Autodesk Inventor part; units mm, degrees
ref_plane "YZ Plane" through (0, 0, 0) normal (1, 0, 0) x (0, 1, 0)
ref_plane "XZ Plane" through (0, 0, 0) normal (0, 1, 0) x (-1, 0, 0)
ref_plane "XY Plane" through (0, 0, 0) normal (0, 0, 1) x (1, 0, 0)
sketch "Sketch1" plane through (0, 0, 0) normal (0, 0, 1) x (1, 0, 0)
  line L0 (-11, 0) -> (11, 0)
  line L1 (11, 0) -> (11, 30)
  line L2 (11, 30) -> (-11, 0)
  point P0 (0, 0)
  point P1 (0, 0)
  dimension "d0" = 22
  dimension "d1" = 30
extrude "Extrusion1" add sketch "Sketch1" along normal mid plane 10
sketch "Sketch2" plane through (0, 0, 0) normal (0, 0, 1) x (1, 0, 0)
  line L0 (11, 30) -> (11, 0) construction
  line L1 (11, 0) -> (-11, 0) construction
  line L2 (-11, 0) -> (11, 30) construction
  line L3 (8.1, 8) -> (0, 8)
  line L4 (0, 8) -> (0, 5)
  line L5 (0, 5) -> (8.1, 5)
  line L6 (8.1, 5) -> (8.1, 8)
  line L7 (6, 11) -> (9, 11)
  line L8 (9, 11) -> (9, 19.1)
  line L9 (9, 19.1) -> (6, 19.1)
  line L10 (6, 19.1) -> (6, 11)
  point P0 (0, 0)
  point P1 (0, 6.5)
  point P2 (0, 0)
  point P3 (11, 15)
  dimension "d4" = 8.1
  dimension "d5" = 5
  dimension "d6" = 3
  dimension "d7" = 3
  dimension "d8" = 8.1
  dimension "d9" = 2
  dimension "d10" = 3
extrude "Extrusion2" cut sketch "Sketch2" along normal through all both and the other way through all
sketch "Sketch3" plane through (11, 0, 5) normal (1, 0, 0) x (0, 0, -1)
  line L0 (10, 19.1) -> (10, 11) construction
  line L1 (10, 19.1) -> (0, 19.1) construction
  line L2 (0, 11) -> (0, 19.1) construction
  line L3 (10, 11) -> (0, 11) construction
  line L4 (10, 19.1) -> (0, 19.1) construction
  line L5 (5, 19.1) -> (5, 11) construction
  line L6 (0, 15.05) -> (10, 15.05) construction
  line L7 (10, 19.1) -> (10, 11) construction
  circle A0 centre (5, 15.05) radius 2.75
  point P0 (5, 0)
  dimension "d13" = 5.5
extrude "Extrusion3" cut sketch "Sketch3" against normal up to surface (5 mm away)
sketch "Sketch4" plane through (-11, 0, 5) normal (0, -1, 0) x (1, 0, 0)
  line L0 (19.1, -10) -> (11, -10) construction
  line L1 (19.1, -10) -> (19.1, 0) construction
  line L2 (11, 0) -> (19.1, 0) construction
  line L3 (11, 0) -> (11, -10) construction
  line L4 (19.1, 0) -> (11, 0) construction
  line L5 (15.05, 0) -> (15.05, -10) construction
  line L6 (19.1, -10) -> (11, -10) construction
  line L7 (11, -5) -> (19.1, -5) construction
  circle A0 centre (15.05, -5) radius 2.75
  dimension "d16" = 5.5
extrude "Extrusion4" cut sketch "Sketch4" against normal up to surface (8 mm away)
properties part number "ligamento_obj4"
Geometry: final body of the model. Coordinates: model frame, mm. A direction names the side the tool comes from. Give positions to 0.01 mm unless a question says otherwise; leave off trailing zeros. Order: outer loops, then holes, each group sorted by start corner. A loop starts at its lowest first (then second) coordinate and runs counter-clockwise, first axis right, second up. Notation, with made-up numbers: (-15.75, -37) - (1.25, -37) arc R12 ccw to (1.25, -22) - close; hole circle Ø4 at (-5, -37). An arc over 180 degrees is marked (long way). Use CSV: the item, a comma, the result in double quotes.
1. Section query C-C (z = 4). Output: boundary loops of the cut face in (x, y), plus the area to 3 significant figures.
Answers below:
outline,"(-11, 0) - (11, 0) - (11, 30) - close; hole (0, 5) - (8.1, 5) - (8.1, 8) - (0, 8) - close; hole (6, 11) - (9, 11) - (9, 19.1) - (6, 19.1) - close"
area,"281 mm2"
2. Access query for faces 5 (the face through (11, 11, 0)), 6 (the face through (4, 8, 0)). Directions: +Z, -Z, +X, -X, +Y, -Y. A direction counts if a zero-diameter tool reaches every point of the face in a straight line with its end or side. Return the directions, or none.
Answers below:
face 5,"+Z, -Z, +X, +Y, -Y"
face 6,"+Z, -Z"
3. Mould query, pull axis Z, two halves, no side actions, for faces 1 (the face through (5, 9, 5)), 2 (the face through (6.59, 2.46, -1.05)), 3 (the face through (10.014, 12.365, 0.596)), 4 (the face through (0, 15, 0)). Classes: +Z half, -Z half, draft (parallel to the pull), parting line (faces both ways), or undercut.
Answers below:
face 1,"+Z half"
face 2,"undercut"
face 3,"undercut"
face 4,"draft"
4. Material intervals for line 1 along Z through (x, y) = (4.05, 1.25); line 2 along Z through (x, y) = (9.5, 13.75); line 3 along Y through (x, z) = (9.7, 0), sorted ascending. Write a range as from..to.
Answers below:
line 1,"-5..-2.75, 2.75..5"
line 2,"-5..-2.42, 2.42..5"
line 3,"0..12.3, 17.8..28.23"
5. Section query D-D (z = 1.25). Output: boundary loops of the cut face in (x, y).
Answers below:
outline,"(-11, 0) - (1.6, 0) - (1.6, 5) - (0, 5) - (0, 8) - (8.1, 8) - (8.1, 5) - (6.5, 5) - (6.5, 0) - (11, 0) - (11, 12.6) - (9, 12.6) - (9, 11) - (6, 11) - (6, 19.1) - (9, 19.1) - (9, 17.5) - (11, 17.5) - (11, 30) - close"
6. Contact query for flat-ended pins moving along their axis: pin 1 (1.5 mm diameter, centred on y = 17.5, z = 3, fed in from -X); pin 2 (4.5 mm diameter, centred on x = 4.05, z = 0, fed in from +Y); pin 3 (6 mm diameter, centred on y = 25.5, z = -2, fed in from -X). Output: stop coordinate, or through.
Answers below:
pin 1,"x = 1.28"
pin 2,"y = 23.59"
pin 3,"x = 5.5"
7. Section query B-B (x = 4.05). Output: boundary loops of the cut face in (y, z), plus the area to 3 significant figures.
Answers below:
outline,"(0, -5) - (5, -5) - (5, -2.75) - (0, -2.75) - close; (0, 2.75) - (5, 2.75) - (5, 5) - (0, 5) - close; (8, -5) - (20.52, -5) - (20.52, 5) - (8, 5) - close"
area,"148 mm2"
8. Section query A-A (y = 15.05). Output: boundary loops of the cut face in (x, z).
Answers below:
outline,"(0.04, -5) - (6, -5) - (6, 5) - (0.04, 5) - close; (9, -5) - (11, -5) - (11, -2.75) - (9, -2.75) - close; (9, 2.75) - (11, 2.75) - (11, 5) - (9, 5) - close"
